```python
from build123d import *

# Parameters (mm, degrees)
SKETCH1_W                = 20
SKETCH1_H                = 100
BOSS_EXTRUDE1_DEPTH      = 200
SKETCH2_W                = 9
SKETCH2_H                = 70
CUT_EXTRUDE1_DEPTH       = 207.397674406
M2_CLEARANCE_HOLE1_D     = 2.4
M2_CLEARANCE_HOLE1_DEPTH = 4
M2_CLEARANCE_HOLE1_TIP   = 0.721032743
M2_CLEARANCE_HOLE2_D     = 2.4
M2_CLEARANCE_HOLE2_DEPTH = 4
M2_CLEARANCE_HOLE2_TIP   = 0.721032743
M2_CLEARANCE_HOLE4_D     = 2.4
SKETCH13_W               = 20
SKETCH13_H               = 26
CUT_EXTRUDE2_DEPTH       = 207.397674406
M2_CLEARANCE_HOLE5_D     = 2.4
M2_CLEARANCE_HOLE5_DEPTH = 11
M2_CLEARANCE_HOLE5_TIP   = 0.721032743
M2_CLEARANCE_HOLE6_D     = 2.4
M2_CLEARANCE_HOLE6_DEPTH = 11
M2_CLEARANCE_HOLE6_TIP   = 0.721032743
M2_CLEARANCE_HOLE7_D     = 2.4
M2_CLEARANCE_HOLE7_DEPTH = 11
M2_CLEARANCE_HOLE7_TIP   = 0.721032743


with BuildPart() as part:
    # Sketch1 → Boss-Extrude1 (new body)
    with BuildSketch(Plane(origin=(0, 0, 0), x_dir=(1, 0, 0), z_dir=(0, 1, 0))):
        Rectangle(SKETCH1_W, SKETCH1_H)
    extrude(amount=BOSS_EXTRUDE1_DEPTH)

    # Sketch2 → Cut-Extrude1 (cut, through all)
    with BuildSketch(Plane(origin=(0, 200, 0), x_dir=(1, 0, 0), z_dir=(0, 1, 0))):
        with Locations((-5.5, -15)):
            Rectangle(SKETCH2_W, SKETCH2_H)
    extrude(amount=-CUT_EXTRUDE1_DEPTH, mode=Mode.SUBTRACT)

    # M2 Clearance Hole1
    with Locations(Plane(origin=(0, 200, 0), x_dir=(1, 0, 0), z_dir=(0, 1, 0))):
        with Locations((4.5, 40), (4.5, -40)):
            Hole(M2_CLEARANCE_HOLE1_D / 2, depth=M2_CLEARANCE_HOLE1_DEPTH)
            with Locations((0, 0, -(M2_CLEARANCE_HOLE1_DEPTH + M2_CLEARANCE_HOLE1_TIP / 2))):  # 118° drill point
                Cone(0, M2_CLEARANCE_HOLE1_D / 2, M2_CLEARANCE_HOLE1_TIP, mode=Mode.SUBTRACT)

    # M2 Clearance Hole2
    with Locations(Plane(origin=(0, 0, 0), x_dir=(-1, 0, 0), z_dir=(0, -1, 0))):
        with Locations((-4.5, 40), (-4.5, -40)):
            Hole(M2_CLEARANCE_HOLE2_D / 2, depth=M2_CLEARANCE_HOLE2_DEPTH)
            with Locations((0, 0, -(M2_CLEARANCE_HOLE2_DEPTH + M2_CLEARANCE_HOLE2_TIP / 2))):  # 118° drill point
                Cone(0, M2_CLEARANCE_HOLE2_D / 2, M2_CLEARANCE_HOLE2_TIP, mode=Mode.SUBTRACT)

    # M2 Clearance Hole4 (through all)
    with Locations(Plane(origin=(0, 0, -50), x_dir=(-1, 0, 0), z_dir=(0, 0, -1))):
        with Locations((5, 190), (5, 10)):
            Hole(M2_CLEARANCE_HOLE4_D / 2)

    # Sketch13 → Cut-Extrude2 (cut, through all)
    with BuildSketch(Plane.XZ):
        with Locations((0, -37)):
            Rectangle(SKETCH13_W, SKETCH13_H)
    extrude(amount=-CUT_EXTRUDE2_DEPTH, mode=Mode.SUBTRACT)

    # M2 Clearance Hole5
    with Locations(Plane(origin=(0, 0, 0), x_dir=(-1, 0, 0), z_dir=(0, -1, 0))):
        with Locations((-4.5, 14)):
            Hole(M2_CLEARANCE_HOLE5_D / 2, depth=M2_CLEARANCE_HOLE5_DEPTH)
            with Locations((0, 0, -(M2_CLEARANCE_HOLE5_DEPTH + M2_CLEARANCE_HOLE5_TIP / 2))):  # 118° drill point
                Cone(0, M2_CLEARANCE_HOLE5_D / 2, M2_CLEARANCE_HOLE5_TIP, mode=Mode.SUBTRACT)

    # M2 Clearance Hole6
    with Locations(Plane(origin=(0, 200, 0), x_dir=(1, 0, 0), z_dir=(0, 1, 0))):
        with Locations((4.5, 14)):
            Hole(M2_CLEARANCE_HOLE6_D / 2, depth=M2_CLEARANCE_HOLE6_DEPTH)
            with Locations((0, 0, -(M2_CLEARANCE_HOLE6_DEPTH + M2_CLEARANCE_HOLE6_TIP / 2))):  # 118° drill point
                Cone(0, M2_CLEARANCE_HOLE6_D / 2, M2_CLEARANCE_HOLE6_TIP, mode=Mode.SUBTRACT)

    # M2 Clearance Hole7
    with Locations(Plane(origin=(10, 0, 0), x_dir=(0, 0, -1), z_dir=(1, 0, 0))):
        with Locations((9, 20), (9, 180), (-35, 100)):
            Hole(M2_CLEARANCE_HOLE7_D / 2, depth=M2_CLEARANCE_HOLE7_DEPTH)
            with Locations((0, 0, -(M2_CLEARANCE_HOLE7_DEPTH + M2_CLEARANCE_HOLE7_TIP / 2))):  # 118° drill point
                Cone(0, M2_CLEARANCE_HOLE7_D / 2, M2_CLEARANCE_HOLE7_TIP, mode=Mode.SUBTRACT)


solid = part.part
```
The model under review builds one solid part; all positions refer to its coordinate system, in mm. A direction names the side the tool comes from. Round coordinates to 2 decimals unless told otherwise and drop trailing zeros. Loops run counter-clockwise (first coordinate to the right, second up) from the corner with the lowest first, then second, coordinate; pieces in that order, holes last.
1) Clearance check with flat-ended pins moving along their axes: P1, Ø6, axis at x = -7.5, y = 130, coming from the +Z side; P2, Ø1.4, axis at x = 4.5, z = -14, coming from the +Y side; P3, Ø1.5, axis at y = 35, z = 28, coming from the -X side. State where each tip first meets the part, or that it passes through.
Values follow:
P1: stops at z = -20
P2: stops at y = 188.7
P3: stops at x = -1
2) Wall thickness on line 1 along Z through (x, y) = (4.5, 2.3); line 2 along X through (y, z) = (198, 40); line 3 along Z through (x, y) = (4.5, 7.25): over which ranges is each line inside the solid? List them lowest first.
Values follow:
line 1: z = -24 to -15.2, -12.8 to 38.8, 41.2 to 50
line 2: x = -1 to 3.3, 5.7 to 10
line 3: z = -24 to -15.2, -12.8 to 50
3) Consider section B-B on z = 28. State the section outline as (x, y) points, then the cut area to 3 significant figures.
Values follow:
outline: (-1, 0) - (10, 0) - (10, 200) - (-1, 200) - close
area: 2,200 mm2
4) Tool access review of faces 1 (the face through (4, 99, 50)), 2 (the face through (-1, 101, 15)): name each direction out of +Z, -Z, +X, -X, +Y, -Y from which nothing blocks a thin tool from reaching the whole face with its end or side.
Values follow:
face 1: +Z, +X, -X, +Y, -Y
face 2: +Z, -X, +Y, -Y
5) Consider section A-A on y = 117. State the section outline as (x, z) points, then the cut area to 3 significant figures.
Values follow:
outline: (-10, -24) - (10, -24) - (10, 50) - (-1, 50) - (-1, -20) - (-10, -20) - close
area: 850 mm2
